from build123d import *

# Parameters (mm, degrees)
F0_W     = 10
F0_H     = 150
F1_DEPTH = 2
F2_W     = 3
F2_H     = 150
F3_DEPTH = 4.5
F4_W     = 3
F4_H     = 150
F4_W_2   = 7
F5_DEPTH = 2
F6_W     = 3
F6_H     = 150
F7_DEPTH = 4.5
F8_W     = 3
F8_H     = 150
F8_W_2   = 7
F9_DEPTH = 2
F10_R    = 2


# Not quite as in the source:
# - a feature names something its author has since deleted; it is built from what else it names


with BuildPart() as f1:
    # F0 (on Top) → F1 (new body)
    with BuildSketch(Plane.XY):
        Rectangle(F0_W, F0_H)
    extrude(amount=F1_DEPTH)

    # F2 (on face) → F3 (join)
    with BuildSketch(Plane.XY.offset(2)):
        with Locations((3.5, 0)):
            Rectangle(F2_W, F2_H)
    extrude(amount=F3_DEPTH)

    # F4 (on face) → F5 (join)
    with BuildSketch(Plane.XY.offset(6.5)):
        with Locations((3.5, 0)):
            Rectangle(F4_W, F4_H)
        with Locations((-1.5, 0)):
            Rectangle(F4_W_2, F4_H)
    extrude(amount=F5_DEPTH)

    # F6 (on face) → F7 (join)
    with BuildSketch(Plane.XY.offset(8.5)):
        with Locations((-3.5, 0)):
            Rectangle(F6_W, F6_H)
    extrude(amount=F7_DEPTH)

    # F8 (on face) → F9 (join)
    with BuildSketch(Plane.XY.offset(13)):
        with Locations((-3.5, 0)):
            Rectangle(F8_W, F8_H)
        with Locations((1.5, 0)):
            Rectangle(F8_W_2, F8_H)
    extrude(amount=F9_DEPTH)

    # F10
    f10_edges = [f1.edges().sort_by_distance(p)[0] for p in [
        (-5, 75, 10.75),
        (5, 75, 4.25),
        (-5, -75, 10.75),
        (5, -75, 4.25),
    ]]
    fillet(f10_edges, radius=F10_R)


solid = f1.part
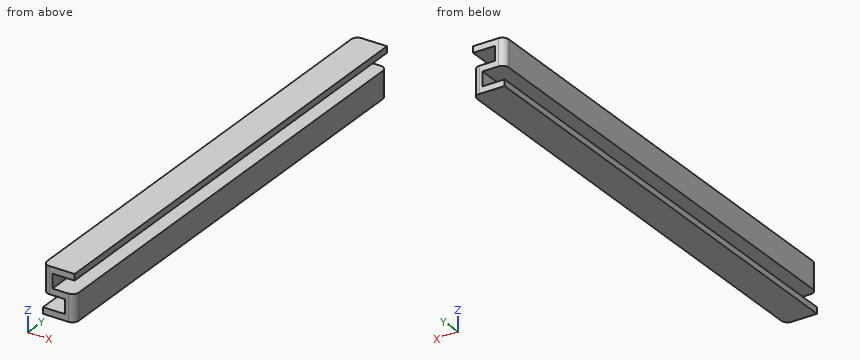
For this review, take the finished solid that the model builds, in its own axes (mm). Round coordinates to 2 decimals unless told otherwise and drop trailing zeros. Loops run counter-clockwise (first coordinate to the right, second up) from the corner with the lowest first, then second, coordinate; pieces in that order, holes last. Notation, with made-up numbers: (-8, -21.5) - (5, -21.5) arc R18 ccw to (5, -10.5) - close; hole circle Ø5 at (2.25, 61). An arc over 180 degrees is marked (long way). Use one line per item in the form item = value.
1) Wall thickness on probe 1 along Z at (x, y) = (0, 32); probe 2 along Z at (x, y) = (-3.75, 53); probe 3 along X at (y, z) = (-63, 11.5): over which ranges is each line inside the solid? List them lowest first.
Solutions:
probe_1 = 0 to 2, 6.5 to 8.5, 13 to 15
probe_2 = 0 to 2, 6.5 to 15
probe_3 = -5 to -2
2) We need section A-A on x = 0. Write out the cut boundary in (y, z), then the cut area to 3 significant figures.
Solutions:
outline = (-75, 0) - (75, 0) - (75, 2) - (-75, 2) - close; (-75, 6.5) - (75, 6.5) - (75, 8.5) - (-75, 8.5) - close; (-75, 13) - (75, 13) - (75, 15) - (-75, 15) - close
area = 900 mm2
3) Clearance check with flat-ended pins moving along their axes: P1, Ø2, axis at y = -27.5, z = 4, coming from the -X side; P2, Ø1.3, axis at y = -35.5, z = 10, coming from the +X side. State where each tip first meets the part, or that it passes through.
Solutions:
P1 = 2
P2 = -2
4) We need section B-B on y = -54. Write out the cut boundary in (x, z), then the cut area to 3 significant figures.
Solutions:
outline = (-5, 0) - (5, 0) - (5, 8.5) - (-2, 8.5) - (-2, 13) - (5, 13) - (5, 15) - (-5, 15) - (-5, 6.5) - (2, 6.5) - (2, 2) - (-5, 2) - close
area = 87.0 mm2
5) We need section C-C on z = 10.5. Write out the cut boundary in (x, y), then the cut area to 3 significant figures.
Solutions:
outline = (-5, -73) arc R2 ccw to (-3, -75) - (-2, -75) - (-2, 75) - (-3, 75) arc R2 ccw to (-5, 73) - close
area = 448 mm2
